Model file for the job. Use its own axes, mm. Give positions to 0.01 mm unless a question says otherwise; leave off trailing zeros. Write each loop counter-clockwise with the first axis right and the second up, starting at its lowest first coordinate (ties: lowest second). Pieces come first, ordered by that corner, then holes. Notation, with made-up numbers: (71.25, 72.25) - (103.25, 72.25) arc R32 cw to (103.25, 107.25) - close; hole circle Ø11 at (-20, 4.5). An arc over 180 degrees is marked (long way). Use CSV: the item, a comma, the result in double quotes.
from build123d import *

# Parameters (mm, degrees)
SKETCH1_W           = 35
SKETCH1_H           = 115
BOSS_EXTRUDE1_DEPTH = 10
SKETCH2_W           = 29
SKETCH2_H           = 4
BOSS_EXTRUDE2_DEPTH = 50
BOSS_EXTRUDE2_TAPER = 1
SKETCH3_RX          = 3.259941838
SKETCH3_RY          = 1.279729234
BOSS_EXTRUDE3_DEPTH = 40


with BuildPart() as part:
    # Sketch1 → Boss-Extrude1 (new body)
    with BuildSketch(Plane(origin=(0, 0, 0), x_dir=(1, 0, 0), z_dir=(0, 1, 0))):
        with Locations((-24.573170732, -22.073170732)):
            Rectangle(SKETCH1_W, SKETCH1_H)
    extrude(amount=BOSS_EXTRUDE1_DEPTH)

    # Sketch2 → Boss-Extrude2 (add)
    with BuildSketch(Plane.XY.offset(79.573170732)):
        with Locations((-24.573170732, 5)):
            Rectangle(SKETCH2_W, SKETCH2_H)
    extrude(amount=BOSS_EXTRUDE2_DEPTH, taper=BOSS_EXTRUDE2_TAPER)

    # Sketch3 → Boss-Extrude3 (add)
    with BuildSketch(Plane(origin=(0, 0, -35.426829268), x_dir=(-1, 0, 0), z_dir=(0, 0, -1))):
        with Locations((24.573170732, 5)):
            Ellipse(SKETCH3_RX, SKETCH3_RY)
    extrude(amount=BOSS_EXTRUDE3_DEPTH)


solid = part.part
(1) Wall check: probe 1 along Z at (x, y) = (-35, 1.25); probe 2 along Z at (x, y) = (-12, 5.25); probe 3 along X at (y, z) = (3.75, 81.5). Give the ranges that are in metal, low to high. Write a range as [from, to].
Checked values:
probe 1,"z = [-35.43, 79.57]"
probe 2,"z = [-35.43, 129.57]"
probe 3,"x = [-39.04, -10.11]"
(2) Saw through at B-B, the plane y = 1.5. List the corners of the cut face in (x, z), then the cut area to 4 significant figures.
Checked values:
outline,"(-42.07, -35.43) - (-7.07, -35.43) - (-7.07, 79.57) - (-42.07, 79.57) - close"
area,"4,025 mm^2"
(3) Flat gauge pins, fed straight in: P1, Ø1.5, axis at x = -17.5, z = 87, coming from the +Y side; P2, Ø5, axis at x = -20, y = 1.5, coming from the -Z side. Where does each tip first touch, or does it go through?
Checked values:
P1,"stops at y = 6.88"
P2,"stops at z = -35.43"
(4) Saw through at A-A, the plane x = -17.5. List the corners of the cut face in (y, z), then the cut area to 3 significant figures.
Checked values:
outline,"(0, -35.43) - (10, -35.43) - (10, 79.57) - (7, 79.57) - (6.13, 129.57) - (3.87, 129.57) - (3, 79.57) - (0, 79.57) - close"
area,"1,310 mm^2"
